Could you check a few things on this drawing? It's one solid part, dimensions in mm from its lowest x, y, z. A direction names the side the tool comes from. Give positions to 0.01 mm unless a question says otherwise; leave off trailing zeros. Loops run counter-clockwise (first coordinate to the right, second up) from the corner with the lowest first, then second, coordinate; pieces in that order, holes last. Notation, with made-up numbers: M -26.75,-6 L -22.75,-6 A22 ccw -22.75,2 Z; hole C 39.5,88.25 d8. An arc over 180 degrees is marked long. Answer as CSV lines item,"result". Start each with the question number.
Item 1: Will these pins go through, and if not, where does the flat tip stop? P1, Ø1.5, axis at x = 11, z = 11.5, coming from the -Y side; P2, Ø9.5, axis at x = 8, z = 4.5, coming from the -Y side; P3, Ø2, axis at x = 43.5, z = 13, coming from the -Y side.
Item 2: I want a section at D-D on y = 23.5. List the corners of the cut face in (x, z) for me, plus the area to 3 significant figures.
Item 3: I want a section at B-B on z = 2.75. List the corners of the cut face in (x, y) for me.
Item 4: If we mould it in two halves opening along X, with no side actions, what happens to the marked faces 6, 7 and 8? For each: released by +X, released by -X, zero draft, split by the parting line, or undercut.
Item 5: I want a section at C-C on x = 36. List the corners of the cut face in (y, z) for me.
Item 6: If I drill on line 1 along X through (y, z) = (40, 9); line 2 along Y through (x, z) = (7.5, 13.75); line 3 along Y through (x, z) = (26.5, 14.75), over which ranges is the centre line in solid material (lowest first)? Write a range as from..to.
Item 7: For the marked faces 1, 2, 3, 4 and 5, which set-ups out of +Z, -Z, +X, -X, +Y, -Y let a thin tool reach every point of the face, with its end or its side?
Item 8: I want a section at A-A on x = 4.25. List the corners of the cut face in (y, z) for me, plus the area to 4 significant figures.
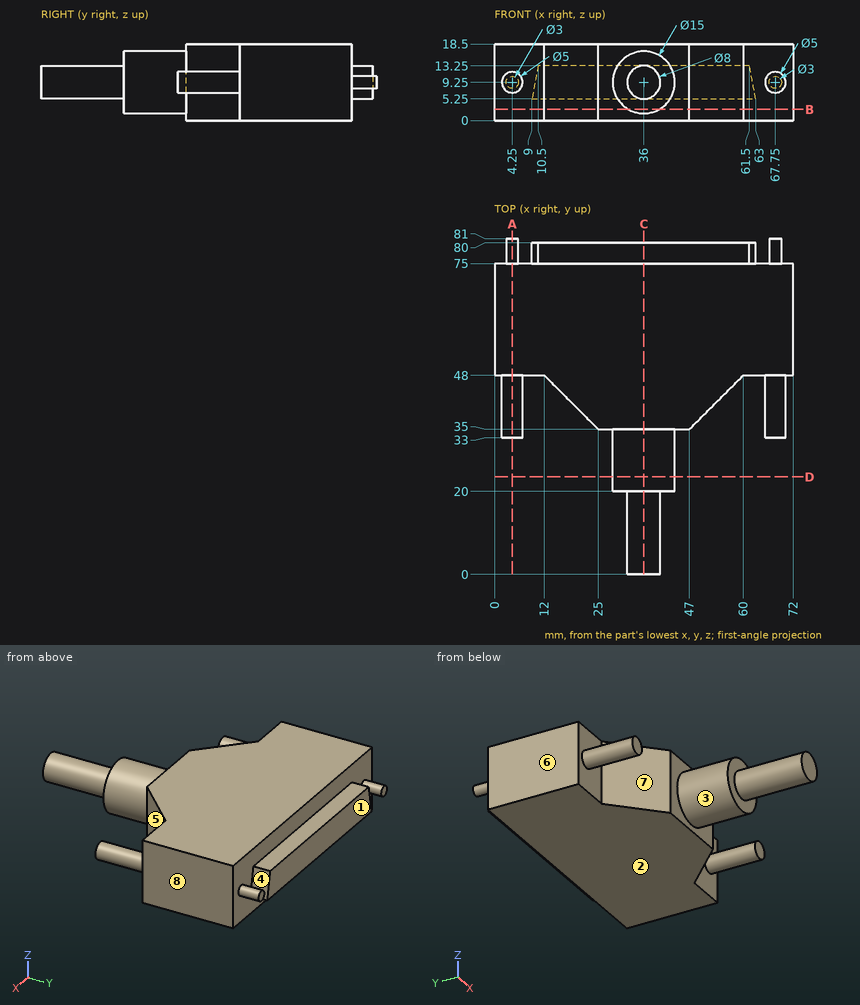
Result:
1,P1,"y = 48"
1,P2,"y = 33"
1,P3,"y = 20"
2,outline,"C 36,9.25 d15"
2,area,"177 mm^2"
3,outline,"M 0,48 L 12,48 L 25,35 L 32.26,35 L 32.26,20 L 39.74,20 L 39.74,35 L 47,35 L 60,48 L 72,48 L 72,75 L 0,75 Z"
4,face 6,"released by -X"
4,face 7,"undercut"
4,face 8,"released by +X"
5,outline,"M 0,5.25 L 20,5.25 L 20,1.75 L 35,1.75 L 35,0 L 75,0 L 75,5.25 L 80,5.25 L 80,13.25 L 75,13.25 L 75,18.5 L 35,18.5 L 35,16.75 L 20,16.75 L 20,13.25 L 0,13.25 Z"
6,line 1,"1.76..6.74, 20..52, 65.26..70.24"
6,line 2,"48..75"
6,line 3,"35..75"
7,face 1,"+Z, -Z, +Y"
7,face 2,"-Z, +X, -X, +Y, -Y"
7,face 3,"-Y"
7,face 4,"+Z, +Y"
7,face 5,"+Z, -Z, -Y"
8,outline,"M 33,6.75 L 48,6.75 L 48,0 L 75,0 L 75,7.75 L 81,7.75 L 81,10.75 L 75,10.75 L 75,18.5 L 48,18.5 L 48,11.75 L 33,11.75 Z"
8,area,"592.5 mm^2"
